The model under review builds one solid part; all positions refer to its coordinate system, in mm. A direction names the side the tool comes from. Give positions to 0.01 mm unless a question says otherwise; leave off trailing zeros. Loops run counter-clockwise (first coordinate to the right, second up) from the corner with the lowest first, then second, coordinate; pieces in that order, holes last. Notation, with made-up numbers: M 80,-30 L 116,-30 A21 ccw 116,-19 Z; hole C -21.5,21.25 d11. An arc over 180 degrees is marked long. Return JSON: item names as keys, results as strings.
```python
from build123d import *

# Parameters (mm, degrees)
CROQUIS1_R              = 2.75
SALIENTE_EXTRUIR1_DEPTH = 5.5


with BuildPart() as part:
    # Croquis1 → Saliente-Extruir1 (new body)
    with BuildSketch(Plane(origin=(0, 0, 0), x_dir=(0, 0, -1), z_dir=(1, 0, 0))):
        with BuildLine():
            Line((-25, 0), (-25, -33.5))
            Line((-25, -33.5), (-25, -39))
            Line((-25, -39), (-5, -39))
            Line((-5, -39), (-5, -33.5))
            Line((-5, -33.5), (5, -33.5))
            Line((5, -33.5), (5, -39))
            Line((5, -39), (25, -39))
            Line((25, -39), (25, -33.5))
            Line((25, -33.5), (25, 0))
            ThreePointArc((25, 0), (16, 9), (7, 0))
            ThreePointArc((7, 0), (0, -7), (-7, 0))
            ThreePointArc((-7, 0), (-16, 9), (-25, 0))
        make_face()
        with Locations((-16, 0)):
            Circle(CROQUIS1_R, mode=Mode.SUBTRACT)
        with Locations((16, 0)):
            Circle(CROQUIS1_R, mode=Mode.SUBTRACT)
    extrude(amount=SALIENTE_EXTRUIR1_DEPTH)


solid = part.part
```
1) Consider section A-A on z = -16. Write out the cut boundary in (x, y), then the cut area to 3 significant figures.
From the geometry:
{"outline": "M 0,-39 L 5.5,-39 L 5.5,-2.75 L 0,-2.75 Z; M 0,2.75 L 5.5,2.75 L 5.5,9 L 0,9 Z", "area": "234 mm²"}
2) Consider section B-B on x = 4.8. Write out the cut boundary in (y, z), then the cut area to 3 significant figures.
From the geometry:
{"outline": "M -39,-25 L 0,-25 A9 ccw 0,-7 A7 cw 0,7 A9 ccw 0,25 L -39,25 L -39,5 L -33.5,5 L -33.5,-5 L -39,-5 Z; hole C 0,-16 d5.5; hole C 0,16 d5.5", "area": "2,020 mm²"}
3) Insertion check: pin 1 (3 mm diameter, centred on x = 1.5, z = -2, fed in from -Y). The pin has a flat end and moves straight along its axis. Give the tip position at first contact, or say it passes through.
From the geometry:
{"pin 1": "y = -33.5"}
4) The part is to be moulded in two halves that separate along Z. For faces 1 (the face through (3, 9, 16)), 2 (the face through (3, -39, 15)), 3 (the face through (3, -19, 25)), 4 (the face through (3, -36, 5)), say which applies: released by +Z, released by -Z, zero draft, split by the parting line, or undercut.
From the geometry:
{"face 1": "undercut", "face 2": "zero draft", "face 3": "released by +Z", "face 4": "undercut"}
5) Wall thickness on L1, parallel to Y at x = 2.85, z = -16; L2, parallel to Z at x = 3.95, y = 1; L3, parallel to Z at x = 2.35, y = 5.5: over which ranges is each line inside the solid? List them lowest first. Write a range as from..to.
From the geometry:
{"L1": "-39..-2.75, 2.75..9", "L2": "-24.94..-18.56, -13.44..-7.06, 7.06..13.44, 18.56..24.94", "L3": "-23.12..-8.88, 8.88..23.12"}
6) Consider section D-D on z = 9. Write out the cut boundary in (x, y).
From the geometry:
{"outline": "M 0,-39 L 5.5,-39 L 5.5,5.66 L 0,5.66 Z"}
7) Consider section C-C on z = 16.5. Write out the cut boundary in (x, y), then the cut area to 3 significant figures.
From the geometry:
{"outline": "M 0,-39 L 5.5,-39 L 5.5,-2.7 L 0,-2.7 Z; M 0,2.7 L 5.5,2.7 L 5.5,8.99 L 0,8.99 Z", "area": "234 mm²"}
8) Tool access review of faces 5 (the face through (3, -36, -5)), 6 (the face through (3, -20, -25)): name each direction out of +Z, -Z, +X, -X, +Y, -Y from which nothing blocks a thin tool from reaching the whole face with its end or side.
From the geometry:
{"face 5": "+X, -X, -Y", "face 6": "-Z, +X, -X, +Y, -Y"}
